from build123d import *

# Parameters (mm, degrees)
F3_DEPTH = 8
F0_R     = 5.1
F4_DEPTH = 25.4
F5_DEPTH = 25.4


with BuildPart() as f3:
    # F2 (on face) → F3 (new body)
    with BuildSketch(Plane.XY):
        Polygon((0.021091, -22.923663), (19.86302, -11.443566), (19.841929, 11.480097), (-0.021091, 22.923663), (-19.86302, 11.443566), (-19.841929, -11.480097), align=None)
    extrude(amount=F3_DEPTH)

    # F0 (on Top) → F4 (cut)
    with BuildSketch(Plane.XY):
        Circle(F0_R)
    extrude(amount=-F4_DEPTH, mode=Mode.SUBTRACT)

    # F0 (on Top) → F5 (cut)
    with BuildSketch(Plane.XY):
        Circle(F0_R)
    extrude(amount=-F5_DEPTH, mode=Mode.SUBTRACT)


solid = f3.part
CAD build for the part. Positions are in the model's coordinates, mm. Round coordinates to 2 decimals unless told otherwise and drop trailing zeros. Write each loop counter-clockwise with the first axis right and the second up, starting at its lowest first coordinate (ties: lowest second). Pieces come first, ordered by that corner, then holes. Notation, with made-up numbers: M -12.75,56 L 38.25,56 A24 ccw 38.25,92 Z; hole C 38.25,76.25 d2. An arc over 180 degrees is marked long. Use a Markdown table: item, result. Add a question column.
1. Slice it at C-C on x = -16.5. Give the cut face in (y, z), then the cut area to 3 significant figures.
2. Flat gauge pins, fed straight in: P1, Ø3, axis at x = 1.5, z = 2.5, coming from the +Y side; P2, Ø1, axis at y = 12, z = 1, coming from the -X side; P3, Ø1, axis at x = 11, z = 6.5, coming from the +Y side. Where does each tip first touch, or does it go through?
3. Slice it at A-A on z = 4.5. Give the cut face in (x, y).
4. Slice it at B-B on y = -14. Give the cut face in (x, z).
5. Drill centre lines: probe 1 along X at (y, z) = (8, 5.5); probe 2 along X at (y, z) = (-2, 2); probe 3 along Y at (x, z) = (0, 0.75). Where is each one in solid material? Low to high.
Reply:
| question | item | result |
|---|---|---|
| 1 | outline | M -13.41,0 L 13.39,0 L 13.39,8 L -13.41,8 Z |
| 1 | area | 214 mm^2 |
| 2 | P1 | stops at y = 22.91 |
| 2 | P2 | stops at x = -19.77 |
| 2 | P3 | stops at y = 16.86 |
| 3 | outline | M -19.86,11.44 L -19.84,-11.48 L 0.02,-22.92 L 19.86,-11.44 L 19.84,11.48 L -0.02,22.92 Z |
| 4 | outline | M -15.47,0 L 15.44,0 L 15.44,8 L -15.47,8 Z |
| 5 | probe 1 | x = -19.86 to 19.85 |
| 5 | probe 2 | x = -19.85 to 19.85 |
| 5 | probe 3 | y = -22.91 to 22.91 |
